The model under review builds one solid part; all positions refer to its coordinate system, in mm. Face numbers are marked on the shaded views. A direction names the side the tool comes from. Round coordinates to 2 decimals unless told otherwise and drop trailing zeros. Write each loop counter-clockwise with the first axis right and the second up, starting at its lowest first coordinate (ties: lowest second). Pieces come first, ordered by that corner, then holes. Notation, with made-up numbers: M -36,40 L -14,40 A27 ccw -14,57 Z; hole C 57.25,-24.5 d7. An arc over 180 degrees is marked long. One line per item, written item: value. Start each with the question number.
1) Wall thickness on probe 1 along Z at (x, y) = (0, 3.9); probe 2 along Y at (x, z) = (15, -13); probe 3 along Z at (x, y) = (28, 20): over which ranges is each line inside the solid? List them lowest first.
2) For P1, Ø4, axis at x = -15, y = 35, coming from the -Z side; P2, Ø11, axis at y = 58, z = -17.5, coming from the -X side; P3, Ø5, axis at x = 15, y = 35, coming from the +Z side, all flat-tipped, find the tip position at first contact; note any pin that passes through.
3) Take a section at B-B, the plane z = 0. Write out the cut boundary in (x, y), and give its area (3 significant figures).
4) Take a section at D-D, the plane x = 15. Write out the cut boundary in (y, z).
5) Take a section at C-C, the plane y = 70. Write out the cut boundary in (x, z), and give its area (3 significant figures).
6) Tool access review of the marked faces 1, 2, 3 and 4: name each direction out of +Z, -Z, +X, -X, +Y, -Y from which nothing blocks a thin tool from reaching the whole face with its end or side.
7) Take a section at A-A, the plane x = 0. Write out the cut boundary in (y, z), and give its area (4 significant figures).
Autodesk Inventor part; units mm, degrees
ref_plane "YZ Plane" through (0, 0, 0) normal (1, 0, 0) x (0, 1, 0)
ref_plane "XZ Plane" through (0, 0, 0) normal (0, 1, 0) x (-1, 0, 0)
ref_plane "XY Plane" through (0, 0, 0) normal (0, 0, 1) x (1, 0, 0)
sketch "Sketch1" plane through (0, 0, 0) normal (0, 1, 0) x (-1, 0, 0)
  circle A0 centre (0, 0) radius 40
  circle A1 centre (0, 0) radius 2.5
  dimension "d0" = 80
  dimension "d1" = 5
extrude "Extrusion1" add sketch "Sketch1" along normal blind 5
sketch "Sketch2" plane through (0, 5, 0) normal (0, 1, 0) x (1, 0, 0)
  line L0 (0, 10) -> (30, 10)
  line L1 (30, 10) -> (30, 20)
  line L2 (30, 20) -> (0, 20)
  line L3 (0, 20) -> (-30, 20)
  line L4 (-30, 20) -> (-30, 10)
  line L5 (-30, 10) -> (0, 10)
  point P0 (0, 0)
  dimension "d5" = 30
  dimension "d6" = 10
extrude "Extrusion2" add sketch "Sketch2" along normal blind 80
sketch "Sketch3" plane through (-30, 5, -10) normal (0, 0, 1) x (1, 0, 0)
  line L0 (60, 80) -> (0, 80)
  circle A0 centre (40, 65) radius 1.5
  circle A1 centre (20, 65) radius 1.5
  line L1 (0, 0) -> (0, 80)
  circle A2 centre (45, 30) radius 1.5
  circle A3 centre (15, 30) radius 1.5
  point P0 (30, -5)
  dimension "d13" = 3
  dimension "d14" = 3
  dimension "d18" = 3
  dimension "d19" = 3
extrude "Extrusion3" cut sketch "Sketch3" against normal blind 5
sketch "Sketch4" plane through (-30, 5, -10) normal (0, 0, 1) x (1, 0, 0)
  point P0 (30, -5)
properties part number "gripper"
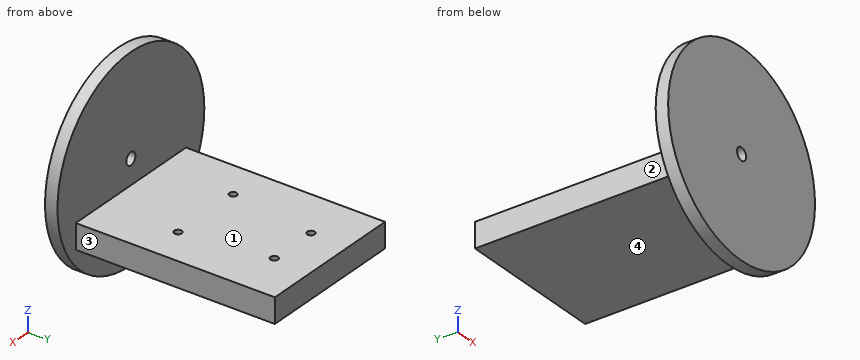
Checked values:
1. probe 1: z = -40 to -2.5, 2.5 to 40
1. probe 2: y = 0 to 33.5, 36.5 to 85
1. probe 3: z = -20 to -10
2. P1: stops at z = -20
2. P2: stops at x = -30
2. P3: stops at z = -10
3. outline: M -40,0 L -2.5,0 L -2.5,5 L -40,5 Z; M 2.5,0 L 40,0 L 40,5 L 2.5,5 Z
3. area: 375 mm2
4. outline: M 0,-37.08 L 5,-37.08 L 5,-20 L 85,-20 L 85,-10 L 36.5,-10 L 36.5,-15 L 33.5,-15 L 33.5,-10 L 5,-10 L 5,37.08 L 0,37.08 Z
5. outline: M -30,-20 L 30,-20 L 30,-10 L 11.5,-10 L 11.5,-15 L 8.5,-15 L 8.5,-10 L -8.5,-10 L -8.5,-15 L -11.5,-15 L -11.5,-10 L -30,-10 Z
5. area: 570 mm2
6. face 1: +Z, +X, -X, +Y
6. face 2: +Z, -Z, -X, +Y
6. face 3: +Z, -Z, +X, +Y
6. face 4: -Z, +X, -X, +Y
7. outline: M 0,-40 L 5,-40 L 5,-20 L 85,-20 L 85,-10 L 5,-10 L 5,-2.5 L 0,-2.5 Z; M 0,2.5 L 5,2.5 L 5,40 L 0,40 Z
7. area: 1,175 mm2
